Input: part model. Units: mm. Frame: model coordinates. Face numbers are marked on the shaded views. A direction names the side the tool comes from. Coordinates: 2 decimals unless noted, no trailing zeros. Loops run counter-clockwise (first coordinate to the right, second up) from the corner with the lowest first, then second, coordinate; pieces in that order, holes last.
Item 1: Contact query for flat-ended pins moving along their axis: P1, Ø5, axis at y = 40.48, z = 0, coming from the -X side; P2, Ø3, axis at y = 14.5, z = 0, coming from the +X side; P3, Ø1.7, axis at x = -22, y = 12.5, coming from the -Z side; P4, Ø1, axis at x = -30.5, z = 0, coming from the -Y side. Output: stop coordinate, or through.
Item 2: Ray query, line 1 along Y through (x, z) = (-2.5, 0); line 2 along Z through (x, y) = (-30, 4); line 3 along X through (y, z) = (6.5, 0). Return the intervals inside material, ascending.
Item 3: Section C-C on y = 14. Return loops of the section in (x, z).
Item 4: Reachability of the marked faces 1, 2, 3, 4 and 5 from +Z, -Z, +X, -X, +Y, -Y: full face, straight path, thin tool, end or side. Return the list, or none.
Item 5: Section B-B on z = 0. Give the number of separate pieces and of enclosed holes in the cut face, and give its area (3 significant figures).
Item 6: Section D-D on x = -35. Return loops of the section in (y, z) (3 decimals).
Item 7: Section A-A on x = -30.48. Return loops of the section in (y, z) (3 decimals).
Autodesk Inventor part; units mm, degrees
ref_plane "YZ Plane" through (0, 0, 0) normal (1, 0, 0) x (0, 1, 0)
ref_plane "XZ Plane" through (0, 0, 0) normal (0, 1, 0) x (-1, 0, 0)
ref_plane "XY Plane" through (0, 0, 0) normal (0, 0, 1) x (1, 0, 0)
sketch "Sketch1" plane through (0, 0, 0) normal (0, 0, 1) x (1, 0, 0)
  line L0 (0, 0) -> (-38.1, 0)
  line L1 (-38.1, 0) -> (-38.1, 9.525)
  line L2 (-38.1, 9.525) -> (-6.35, 9.525)
  line L3 (-6.35, 9.525) -> (-6.35, 50.8)
  line L4 (-6.35, 50.8) -> (0, 50.8)
  line L5 (0, 50.8) -> (0, 0)
  dimension "d0" = 38.1
  dimension "d1" = 9.525
  dimension "d2" = 50.8
  dimension "d3" = 6.35
extrude "Extrusion1" add sketch "Sketch1" along normal mid plane 12.7
sketch "Sketch2" plane through (-6.35, 9.525, 6.35) normal (-1, 0, 0) x (0, 0, 1)
  line L0 (-12.7, 41.275) -> (0, 41.275) construction
  line L1 (-6.35, 41.275) -> (-6.35, 0) construction
  line L2 (-12.7, 0) -> (0, 0) construction
  point P0 (-6.35, -9.525)
  point P1 (-6.35, 30.9563)
  point P2 (-6.35, 10.3188)
  dimension "d6" = 10.3187
  dimension "d7" = 10.3187
hole "Hole1" at (-6.35, 40.4812, 0) at (-6.35, 19.8438, 0) direction (1, 0, 0) diameter 3.81 end through all countersink diameter 7.0866 countersink angle 82
sketch "Sketch3" plane through (-38.1, 0, 6.35) normal (0, -1, 0) x (1, 0, 0)
  line L0 (38.1, -6.35) -> (0, -6.35) construction
  line L1 (0, -12.7) -> (0, 0) construction
  line L2 (38.1, -12.7) -> (38.1, 0)
  point P0 (7.62, -6.35)
  dimension "d15" = 30.48
hole "Hole2" at (-30.48, 0, 0) direction (0, 1, 0) diameter 3.302 depth 8.89
fillet "FilletForTop" radius 2.54 4 edges at (-6.35, 50.8, 0) (-3.175, 50.8, 6.35) (0, 50.8, 0) (-3.175, 50.8, -6.35)
fillet "FilletForFront" radius 2.54 8 edges at (-5.6061, 50.0561, -5.6061) (-6.35, 28.8925, -6.35) (-5.6061, 50.0561, 5.6061) (-6.35, 28.8925, 6.35) (-6.35, 9.525, 0) (-38.1, 9.525, 0) (-22.225, 9.525, 6.35) (-22.225, 9.525, -6.35)
sketch "Sketch4" plane through (0, 0, 0) normal (0, 0, 1) x (1, 0, 0)
  line L0 (-6.35, 48.26) -> (-6.35, 12.065)
  line L1 (-8.89, 9.525) -> (-35.56, 9.525)
  line L2 (-6.35, 15.0304) -> (-27.559, 9.525)
  line L3 (-4.4654, 17.9387) -> (-6.35, 16.3004)
  line L4 (-28.829, 8.89) -> (-28.829, 0)
  line L5 (-6.35, 15.0304) -> (-6.35, 9.525)
  line L6 (-6.35, 9.525) -> (-27.559, 9.525)
  point P0 (0, 0)
  point P1 (-6.35, 12.065)
  dimension "d26" = 1.27
  dimension "d27" = 1.27
extrude "Extrusion2" add sketch "Sketch4" along normal mid plane 3.175
equation "\"d0\" = distanceFromWall"
equation "\"d1\" = baseThickness"
equation "\"d2\" = wallHeight"
equation "\"d3\" = wallThickness"
equation "\"d4\" = width"
equation "\"d28\" = 0.25 * width"
equation "\"baseThickness\" = 9.525"
equation "\"wallThickness\" = 6.35"
equation "\"distanceFromWall\" = 38.1"
equation "\"wallHeight\" = 50.8"
equation "\"width\" = 12.7"
equation "\"baseHeight\" = wallHeight - baseThickness"
equation "\"wallHoleCentersDistanceFromEnd\" = 0.25 * baseHeight"
equation "\"lightHoleDistanceFromWall\" = 30.48"
equation "\"screwDepth\" = 7.62"
properties part number "LightLBracket" material "PC/ABS Plastic"
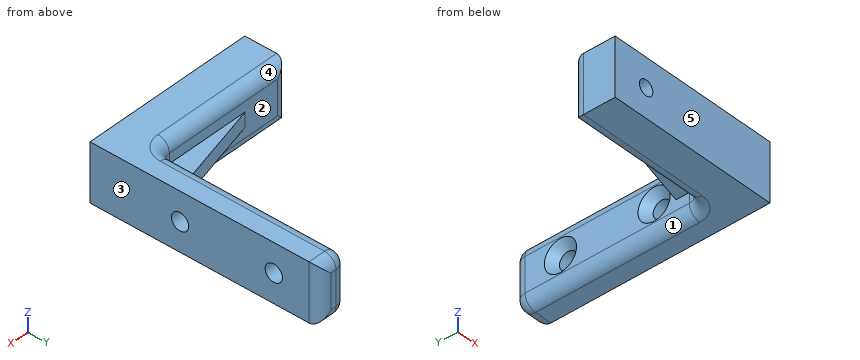
Results found:
1. P1: stops at x = -5.15
1. P2: stops at x = 0
1. P3: passes through
1. P4: stops at y = 8.89
2. line 1: y = 0 to 17.94, 21.75 to 38.58, 42.39 to 50.8
2. line 2: z = -6.35 to -1.58, 1.58 to 6.35
2. line 3: x = -38.1 to -32.13, -28.83 to 0
3. outline: (-10.32, -1.59) - (-6.35, -1.59) - (-6.35, -3.81) arc R2.54 ccw to (-3.81, -6.35) - (0, -6.35) - (0, 6.35) - (-3.81, 6.35) arc R2.54 ccw to (-6.35, 3.81) - (-6.35, 1.59) - (-10.32, 1.59) - close
4. face 1: -Z, -X, +Y
4. face 2: -X, +Y
4. face 3: +Z, -Z, +X, +Y, -Y
4. face 4: +Z, -X, +Y
4. face 5: +Z, -Z, +X, -X, -Y
5. separate pieces: 3
5. enclosed holes: 0
5. area: 595 mm2
6. outline: (0, -6.35) - (6.985, -6.35) arc R2.54 ccw to (9.525, -3.81) - (9.525, 3.81) arc R2.54 ccw to (6.985, 6.35) - (0, 6.35) - close
7. outline: (0, -6.35) - (6.985, -6.35) arc R2.54 ccw to (9.525, -3.81) - (9.525, 3.81) arc R2.54 ccw to (6.985, 6.35) - (0, 6.35) - (0, 1.651) - (8.89, 1.651) - (8.89, -1.651) - (0, -1.651) - close
